```python
from build123d import *

# Parameters (mm, degrees)
BOSS_EXTRUDE2_DEPTH            = 1.625
SKETCH4_W                      = 3.25
SKETCH4_H                      = 3.5
BOSS_EXTRUDE3_DEPTH            = 0.75
CHAMFER1_SIZE                  = 1
F_1_25_1_25_DIAMETER_HOLE1_D   = 1.25
F_1_5_1_5_DIAMETER_HOLE1_D     = 1.5
F_1_5_1_5_DIAMETER_HOLE1_DEPTH = 0.75
F_0_75_0_75_DIAMETER_HOLE1_D   = 0.75


with BuildPart() as part:
    # Sketch3 → Boss-Extrude2 (new, symmetric)
    with BuildSketch(Plane.XY):
        with BuildLine():
            Line((0, 1.25), (-3.3875, 1.25))
            Line((-3.3875, 1.25), (-3.3875, 0.5))
            Line((-3.3875, 0.5), (-1.145643924, 0.5))
            ThreePointArc((-1.145643924, 0.5), (-1.045825033, -0.684653197), (0, -1.25))
            Line((0, -1.25), (3.75, -1.25))
            Line((3.75, -1.25), (3.75, -0.5))
            Line((3.75, -0.5), (1.145643924, -0.5))
            ThreePointArc((1.145643924, -0.5), (1.045825033, 0.684653197), (0, 1.25))
        make_face()
    extrude(amount=BOSS_EXTRUDE2_DEPTH, both=True)

    # Sketch4 → Boss-Extrude3 (add)
    with BuildSketch(Plane(origin=(3.75, 0, 0), x_dir=(0, 0, -1), z_dir=(1, 0, 0))):
        with Locations((0, 0.5)):
            Rectangle(SKETCH4_W, SKETCH4_H)
    extrude(amount=-BOSS_EXTRUDE3_DEPTH)

    # Chamfer1
    chamfer1_edges = [part.edges().sort_by_distance(p)[0] for p in [
        (3.375, 2.25, -1.625),
        (3.375, 2.25, 1.625),
    ]]
    chamfer(chamfer1_edges, length=CHAMFER1_SIZE)

    # Ø1.25 (1.25) Diameter Hole1 (through all)
    with Locations(Plane.XY.offset(1.625)):
        with Locations((0, 0)):
            Hole(F_1_25_1_25_DIAMETER_HOLE1_D / 2)

    # Ø1.5 (1.5) Diameter Hole1
    with Locations(Plane(origin=(3.75, 0, 0), x_dir=(0, 0, -1), z_dir=(1, 0, 0))):
        with Locations((0, 0.75)):
            Hole(F_1_5_1_5_DIAMETER_HOLE1_D / 2, depth=F_1_5_1_5_DIAMETER_HOLE1_DEPTH)

    # Ø0.75 (0.75) Diameter Hole1 (through all)
    with Locations(Plane(origin=(0, 1.25, 0), x_dir=(1, 0, 0), z_dir=(0, 1, 0))):
        with Locations((-2.25, 0.875)):
            f_0_75_0_75_diameter_hole1 = Hole(F_0_75_0_75_DIAMETER_HOLE1_D / 2)

    # Mirror1: Ø0.75 (0.75) Diameter Hole1 across plane
    add(f_0_75_0_75_diameter_hole1.mirror(Plane.XY), mode=Mode.SUBTRACT)


solid = part.part
```
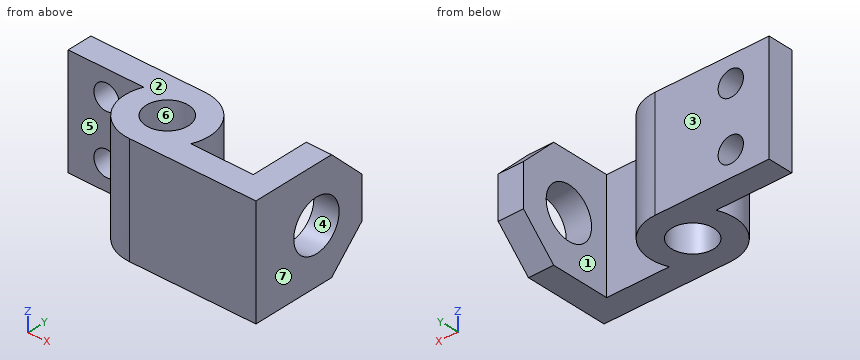
Can you work these out from the model? Positions are in its coordinate system, mm. Face numbers are marked on the shaded views. A direction names the side the tool comes from. Round coordinates to 2 decimals unless told otherwise and drop trailing zeros. Loops run counter-clockwise (first coordinate to the right, second up) from the corner with the lowest first, then second, coordinate; pieces in that order, holes last.
Item 1: Suppose I cut it at A-A, the plane z = 0. State how many separate pieces and enclosed holes the cut face has, then the cut area to 3 significant figures.
Item 2: Please list where these lines run through material, in increasing order: L1, parallel to Y at x = 3.45, z = 0; L2, parallel to Z at x = -2.25, y = 0.7 (3 decimals); L3, parallel to X at y = 0.4, z = 0.85.
Item 3: Will these pins go through, and if not, where does the flat tip stop? pin 1 Ø1 at (x, z) = (-2.5, -0.5) entering from +Y; pin 2 Ø1.5 at (x, z) = (1.5, -1) entering from +Y; pin 3 Ø0.7 at (x, z) = (-2, 0) entering from -Y.
Item 4: Which directions (+Z, -Z, +X, -X, +Y, -Y) give clear straight access to the entire face, cutting with the end or side of a thin tool? Please do the marked faces 1, 2, 3 and 4.
Item 5: If we mould it in two halves opening along X, with no side actions, what happens to the marked faces 5, 6 and 7? For each: +X half, -X half, draft (parallel to the pull), parting line (faces both ways), or undercut.
Item 6: Suppose I cut it at B-B, the plane x = -2.25. Write out the boundary of the cut face in (y, z) (3 decimals).
Item 7: Suppose I cut it at D-D, the plane y = -0.4. Write out the boundary of the cut face in (x, z) (3 decimals), then the cut area to 3 significant figures.
Reported:
1. separate pieces: 2
1. enclosed holes: 1
1. area: 8.73 mm2
2. L1: y = -1.25 to 0, 1.5 to 2.25
2. L2: z = -1.625 to -1.25, -0.5 to 0.5, 1.25 to 1.625
2. L3: x = -1.18 to -0.48, 0.48 to 1.18, 3 to 3.75
3. pin 1: stops at y = 1.25
3. pin 2: stops at y = 1
3. pin 3: stops at y = 0.5
4. face 1: +Z, -Z, +Y
4. face 2: +Z, +X, -X, +Y, -Y
4. face 3: +Z, -Z, -X, +Y
4. face 4: +X
5. face 5: draft
5. face 6: undercut
5. face 7: +X half
6. outline: (0.5, -1.625) - (1.25, -1.625) - (1.25, -1.25) - (0.5, -1.25) - close; (0.5, -0.5) - (1.25, -0.5) - (1.25, 0.5) - (0.5, 0.5) - close; (0.5, 1.25) - (1.25, 1.25) - (1.25, 1.625) - (0.5, 1.625) - close
7. outline: (-1.184, -1.625) - (-0.48, -1.625) - (-0.48, 1.625) - (-1.184, 1.625) - close; (0.48, -1.625) - (1.184, -1.625) - (1.184, 1.625) - (0.48, 1.625) - close; (3, -1.625) - (3.75, -1.625) - (3.75, 1.625) - (3, 1.625) - close
7. area: 7.01 mm2
